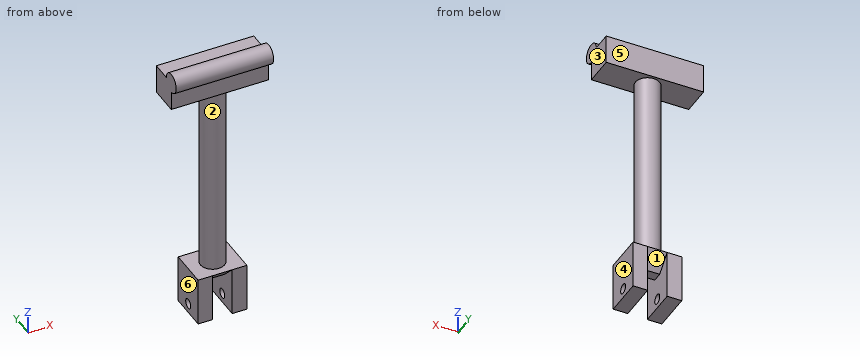
```python
from build123d import *

# Parameters (mm, degrees)
SKIZZE1_W                       = 100
SKIZZE1_H                       = 30
AUFSATZ_LINEAR_AUSTRAGEN1_DEPTH = 30
SKIZZE2_R                       = 10
AUFSATZ_LINEAR_AUSTRAGEN2_DEPTH = 100
SKIZZE3_R                       = 12.5
AUFSATZ_LINEAR_AUSTRAGEN3_DEPTH = 200
SKIZZE4_W                       = 50
SKIZZE4_H                       = 40
AUFSATZ_LINEAR_AUSTRAGEN4_DEPTH = 50
SKIZZE6_W                       = 20
SKIZZE6_H                       = 70
SCHNITT_LINEAR_AUSTRAGEN2_DEPTH = 35
FASE1_SIZE                      = 15
SKIZZE7_R                       = 5
SCHNITT_LINEAR_AUSTRAGEN3_DEPTH = 54


with BuildPart() as part:
    # Skizze1 → Aufsatz-Linear austragen1 (new body)
    with BuildSketch(Plane(origin=(0, 0, 0), x_dir=(1, 0, 0), z_dir=(0, 1, 0))):
        Rectangle(SKIZZE1_W, SKIZZE1_H)
    extrude(amount=AUFSATZ_LINEAR_AUSTRAGEN1_DEPTH)

    # Skizze2 → Aufsatz-Linear austragen2 (add)
    with BuildSketch(Plane(origin=(50, 0, 0), x_dir=(0, 0, -1), z_dir=(1, 0, 0))):
        with Locations((-15, 0)):
            Circle(SKIZZE2_R)
    extrude(amount=-AUFSATZ_LINEAR_AUSTRAGEN2_DEPTH)

    # Skizze3 → Aufsatz-Linear austragen3 (add)
    with BuildSketch(Plane(origin=(0, 0, -15), x_dir=(-1, 0, 0), z_dir=(0, 0, -1))):
        with Locations(Location((0, 15, 0), (0, 0, 180))):
            Circle(SKIZZE3_R)
    extrude(amount=AUFSATZ_LINEAR_AUSTRAGEN3_DEPTH)

    # Skizze4 → Aufsatz-Linear austragen4 (add)
    with BuildSketch(Plane(origin=(0, 0, -215), x_dir=(-1, 0, 0), z_dir=(0, 0, -1))):
        with Locations((0, 15)):
            Rectangle(SKIZZE4_W, SKIZZE4_H)
    extrude(amount=AUFSATZ_LINEAR_AUSTRAGEN4_DEPTH)

    # Skizze6 → Schnitt-Linear austragen2 (cut)
    with BuildSketch(Plane(origin=(0, 0, -265), x_dir=(-1, 0, 0), z_dir=(0, 0, -1))):
        Rectangle(SKIZZE6_W, SKIZZE6_H)
    extrude(amount=-SCHNITT_LINEAR_AUSTRAGEN2_DEPTH, mode=Mode.SUBTRACT)

    # Fase1
    fase1_edges = [part.edges().sort_by_distance(p)[0] for p in [
        (0, -5, -230),
        (0, 35, -230),
    ]]
    chamfer(fase1_edges, length=FASE1_SIZE - 0.0001)  # a hair under: the kernel refuses the full size

    # Skizze7 → Schnitt-Linear austragen3 (cut)
    with BuildSketch(Plane(origin=(25, 0, 0), x_dir=(0, 0, -1), z_dir=(1, 0, 0))):
        with Locations(Location((255, 15, 0), (0, 0, 90))):
            Circle(SKIZZE7_R)
    extrude(amount=-SCHNITT_LINEAR_AUSTRAGEN3_DEPTH, mode=Mode.SUBTRACT)


solid = part.part
```
CAD build for the part. Positions are in the model's coordinates, mm. Face numbers are marked on the shaded views. A direction names the side the tool comes from. Give positions to 0.01 mm unless a question says otherwise; leave off trailing zeros. Write each loop counter-clockwise with the first axis right and the second up, starting at its lowest first coordinate (ties: lowest second). Pieces come first, ordered by that corner, then holes. Notation, with made-up numbers: M -16.75,37 L 6.25,37 A38 ccw 6.25,75 Z; hole C -0.75,20 d6. An arc over 180 degrees is marked long. Return JSON: item names as keys, results as strings. Group by question number.
(1) Band-saw the part on B-B (y = 15). Give the cut face in (x, z), and give its area (3 significant figures).
(2) Band-saw the part on D-D (z = -28). Give the cut face in (x, y).
(3) Drill centre lines: L1, parallel to Z at x = -19.75, y = 15; L2, parallel to Z at x = -23.5, y = 11; L3, parallel to X at y = 25.5, z = -227.5. Where is each one in solid material? Low to high. Write a range as [from, to].
(4) Flat gauge pins, fed straight in: pin 1 Ø5 at (y, z) = (3.5, -69) entering from -X; pin 2 Ø2 at (x, z) = (-10.5, -118) entering from -Y; pin 3 Ø3 at (x, y) = (2.5, 14) entering from -Z; pin 4 Ø24 at (x, y) = (2.5, 18.5) entering from -Z. Where does each tip first touch, or does it go through?
(5) Band-saw the part on A-A (z = -246). Give the cut face in (x, y), and give its area (3 significant figures).
(6) 3-axis set-ups, long thin cutter, end or side, ignore diameter. For the marked faces 4, 5 and 6: which of +Z, -Z, +X, -X, +Y, -Y reach the whole face in a straight line?
(7) Mould opens along Z. For the marked faces 1, 2 and 3 say: pulls with the +Z half, pulls with the -Z half, needs draft (parallel to the pull), parting line crosses it, or undercut.
Entries:
{
 "1": {"outline": "M -50,-15 L -12.5,-15 L -12.5,-215 L -25,-215 L -25,-250 L -10,-250 L -10,-230 L 10,-230 L 10,-250 L 25,-250 L 25,-215 L 12.5,-215 L 12.5,-15 L 50,-15 L 50,15 L -50,15 Z; M -25,-265 L -10,-265 L -10,-260 L -25,-260 Z; M 10,-265 L 25,-265 L 25,-260 L 10,-260 Z", "area": "9,500 mm^2"},
 "2": {"outline": "C 0,15 d25"},
 "3": {"L1": "z = [-265, -260], [-250, -215], [-15, 15]", "L2": "z = [-265, -258], [-252, -215], [-15, 15]", "L3": "x = [-25, -10], [10, 25]"},
 "4": {"pin 1": "stops at x = -8.67", "pin 2": "stops at y = 6.88", "pin 3": "stops at z = -230", "pin 4": "stops at z = -265"},
 "5": {"outline": "M -25,-5 L -10,-5 L -10,35 L -25,35 Z; M 10,-5 L 25,-5 L 25,35 L 10,35 Z", "area": "1,200 mm^2"},
 "6": {"face 4": "-Z, +X, +Y, -Y", "face 5": "+Z, +X, -X, +Y", "face 6": "-Z, -X, +Y, -Y"},
 "7": {"face 1": "pulls with the -Z half", "face 2": "undercut", "face 3": "needs draft"}
}
